```python
from build123d import *

# Parameters (mm, degrees)
BOSS_EXTRUDE1_DEPTH = 10.2
BOSS_EXTRUDE2_DEPTH = 1.2
BOSS_EXTRUDE3_DEPTH = 5
FILLET1_R           = 0.8
CUT_EXTRUDE3_REACH  = 70.238
LPATTERN1_COUNT     = 7
LPATTERN1_PITCH     = 4.4
LPATTERN1_COL_COUNT = 7
LPATTERN1_COL_PITCH = 4.4


with BuildPart() as part:
    # Sketch1 → Boss-Extrude1 (new body)
    with BuildSketch(Plane.XY):
        with BuildLine():
            Line((-21.6, 8), (-21.6, 57))
            ThreePointArc((-21.6, 57), (-19.520458146, 62.020458146), (-14.5, 64.1))
            Line((-14.5, 64.1), (14.5, 64.1))
            ThreePointArc((14.5, 64.1), (19.520458146, 62.020458146), (21.6, 57))
            Line((21.6, 57), (21.6, 8))
            ThreePointArc((21.6, 8), (19.520458146, 2.979541854), (14.5, 0.9))
            Line((14.5, 0.9), (-14.5, 0.9))
            ThreePointArc((-14.5, 0.9), (-19.520458146, 2.979541854), (-21.6, 8))
        make_face()
        with BuildLine():
            Line((-20.8, 8), (-20.8, 57))
            ThreePointArc((-20.8, 57), (-18.954772721, 61.454772721), (-14.5, 63.3))
            Line((-14.5, 63.3), (14.5, 63.3))
            ThreePointArc((14.5, 63.3), (18.954772721, 61.454772721), (20.8, 57))
            Line((20.8, 57), (20.8, 8))
            ThreePointArc((20.8, 8), (18.954772721, 3.545227279), (14.5, 1.7))
            Line((14.5, 1.7), (-14.5, 1.7))
            ThreePointArc((-14.5, 1.7), (-18.954772721, 3.545227279), (-20.8, 8))
        make_face(mode=Mode.SUBTRACT)
    extrude(amount=BOSS_EXTRUDE1_DEPTH)

    # Sketch2 → Boss-Extrude2 (add)
    with BuildSketch(Plane(origin=(0, 0, 0), x_dir=(-1, 0, 0), z_dir=(0, 0, -1))):
        with BuildLine():
            Line((-14.5, 63.3), (14.5, 63.3))
            ThreePointArc((14.5, 63.3), (18.954772721, 61.454772721), (20.8, 57))
            Line((20.8, 57), (20.8, 8))
            ThreePointArc((20.8, 8), (18.954772721, 3.545227279), (14.5, 1.7))
            Line((14.5, 1.7), (-14.5, 1.7))
            ThreePointArc((-14.5, 1.7), (-18.954772721, 3.545227279), (-20.8, 8))
            Line((-20.8, 8), (-20.8, 57))
            ThreePointArc((-20.8, 57), (-18.954772721, 61.454772721), (-14.5, 63.3))
        make_face()
    extrude(amount=-BOSS_EXTRUDE2_DEPTH)

    # Sketch3 → Boss-Extrude3 (add)
    with BuildSketch(Plane.XY.offset(1.2)):
        with BuildLine():
            Line((14.5, 1.7), (-14.5, 1.7))
            ThreePointArc((-14.5, 1.7), (-18.954772721, 3.545227279), (-20.8, 8))
            Line((-20.8, 8), (-20.8, 57))
            ThreePointArc((-20.8, 57), (-18.954772721, 61.454772721), (-14.5, 63.3))
            Line((-14.5, 63.3), (14.5, 63.3))
            ThreePointArc((14.5, 63.3), (18.954772721, 61.454772721), (20.8, 57))
            Line((20.8, 57), (20.8, 8))
            ThreePointArc((20.8, 8), (18.954772721, 3.545227279), (14.5, 1.7))
        make_face()
        with BuildLine():
            Line((-14.5, 4.1), (14.5, 4.1))
            ThreePointArc((14.5, 4.1), (17.257716447, 5.242283553), (18.4, 8))
            Line((18.4, 8), (18.4, 57))
            ThreePointArc((18.4, 57), (17.257716447, 59.757716447), (14.5, 60.9))
            Line((14.5, 60.9), (-14.5, 60.9))
            ThreePointArc((-14.5, 60.9), (-17.257716447, 59.757716447), (-18.4, 57))
            Line((-18.4, 57), (-18.4, 8))
            ThreePointArc((-18.4, 8), (-17.257716447, 5.242283553), (-14.5, 4.1))
        make_face(mode=Mode.SUBTRACT)
    extrude(amount=BOSS_EXTRUDE3_DEPTH)

    # Fillet1
    fillet1_edges = [part.edges().sort_by_distance(p)[0] for p in [
        (-17.257716447, 59.757716447, 6.2),
        (-18.4, 32.5, 6.2),
        (18.954772721, 3.545227279, 6.2),
        (20.8, 32.5, 6.2),
        (18.954772721, 61.454772721, 6.2),
        (0, 63.3, 6.2),
        (-18.954772721, 61.454772721, 6.2),
        (-20.8, 32.5, 6.2),
        (-18.954772721, 3.545227279, 6.2),
        (0, 1.7, 6.2),
        (-17.257716447, 5.242283553, 6.2),
        (0, 4.1, 6.2),
        (17.257716447, 5.242283553, 6.2),
        (18.4, 32.5, 6.2),
        (17.257716447, 59.757716447, 6.2),
        (0, 60.9, 6.2),
    ]]
    fillet(fillet1_edges, radius=FILLET1_R)

    # Sketch6 → Cut-Extrude3 (cut, up to next)
    with BuildSketch(Plane.XY.offset(1.2), mode=Mode.PRIVATE) as cut_extrude3_sk1:
        with BuildLine():
            Line((-15, 33.9), (15, 33.9))
            ThreePointArc((15, 33.9), (16.4, 32.5), (15, 31.1))
            Line((15, 31.1), (-15, 31.1))
            ThreePointArc((-15, 31.1), (-16.4, 32.5), (-15, 33.9))
        make_face()
    cut_extrude3_tool1 = extrude(cut_extrude3_sk1.sketch, amount=-CUT_EXTRUDE3_REACH, mode=Mode.PRIVATE) & part.part
    cut_extrude3 = cut_extrude3_tool1.solids().sort_by_distance((0, 32.5, 1.2))[0]
    add(cut_extrude3, mode=Mode.SUBTRACT)

    # LPattern1: Cut-Extrude3 ×7
    with Locations(*[(0, -i * LPATTERN1_PITCH, 0) for i in range(1, LPATTERN1_COUNT)]):
        add(cut_extrude3, mode=Mode.SUBTRACT)

    # LPattern1 col: Cut-Extrude3 ×7
    with Locations(*[(0, i * LPATTERN1_COL_PITCH, 0) for i in range(1, LPATTERN1_COL_COUNT)]):
        add(cut_extrude3, mode=Mode.SUBTRACT)


solid = part.part
```
Here's how the part is built. I have some questions about the finished solid (model axes, mm). A direction names the side the tool comes from. Give positions to 0.01 mm unless a question says otherwise; leave off trailing zeros. Loops run counter-clockwise (first coordinate to the right, second up) from the corner with the lowest first, then second, coordinate; pieces in that order, holes last. Notation, with made-up numbers: M 29.25,26.5 L 84.25,26.5 A12 ccw 84.25,36.5 Z; hole C -6,56.25 d3. An arc over 180 degrees is marked long. Use one line per item in the form item = value. Start each with the question number.
Q1. Will this pin go through, and if not, where does the flat tip stop? pin 1 Ø11 at (x, y) = (1.5, 20.5) entering from +Z.
Q2. If we section it at A-A (z = 3.75): Write out the boundary of the cut face in (x, y), then the cut area to 3 significant figures.
Q3. I need wall thicknesses on line 1 along X through (y, z) = (29.5, 4.75); line 2 along Y through (x, z) = (-0.5, 7.25); line 3 along Y through (x, z) = (9.5, 2). Which ranges of each line are inside material? Lowest first, please.
Q4. Which directions (+Z, -Z, +X, -X, +Y, -Y) give clear straight access to the entire face, cutting with the end or side of a thin tool? Please do faces 1 (the flat face through (0, 31.1, 1)), 2 (the flat face through (0, 4.1, 3)).
Q5. If we section it at C-C (x = -3): State how many separate pieces and enclosed holes the cut face has, then the cut area to 3 significant figures.
Q6. If we section it at B-B (y = 28.1): Write out the boundary of the cut face in (x, z), then the cut area to 3 significant figures.
Taken from the geometry:
q1.pin_1 = 1.2
q2.outline = M -21.6,8 A7.1 ccw -14.5,0.9 L 14.5,0.9 A7.1 ccw 21.6,8 L 21.6,57 A7.1 ccw 14.5,64.1 L -14.5,64.1 A7.1 ccw -21.6,57 Z; hole M -18.4,8 A3.9 ccw -14.5,4.1 L 14.5,4.1 A3.9 ccw 18.4,8 L 18.4,57 A3.9 ccw 14.5,60.9 L -14.5,60.9 A3.9 ccw -18.4,57 Z
q2.area = 610 mm^2
q3.line_1 = -21.6 to -18.4, 18.4 to 21.6
q3.line_2 = 0.9 to 1.7, 63.3 to 64.1
q3.line_3 = 0.9 to 4.1, 60.9 to 64.1
q4.face_1 = +Z, -Z
q4.face_2 = +Z
q5.separate_pieces = 14
q5.enclosed_holes = 0
q5.area = 70.6 mm^2
q6.outline = M -21.6,0 L -16.4,0 L -16.4,1.2 L -18.4,1.2 L -18.4,5.4 A0.8 ccw -19.2,6.2 L -20,6.2 A0.8 cw -20.8,7 L -20.8,10.2 L -21.6,10.2 Z; M 16.4,0 L 21.6,0 L 21.6,10.2 L 20.8,10.2 L 20.8,7 A0.8 cw 20,6.2 L 19.2,6.2 A0.8 ccw 18.4,5.4 L 18.4,1.2 L 16.4,1.2 Z
q6.area = 50.9 mm^2
